from build123d import *

# Parameters (mm, degrees)
F1_DEPTH = 19
F3_DEPTH = 4


with BuildPart() as f1:
    # F0 (on Right) → F1 (new body)
    with BuildSketch(Plane.YZ):
        Polygon((6.931424, 163.453436), (-53.068576, 163.453436), (-115.068576, 5.453436), (-115.068576, -134.546564), (68.931424, -134.546564), (68.931424, 5.453436), align=None)
    extrude(amount=F1_DEPTH)

    # F2 (on face) → F3 (cut)
    with BuildSketch(Plane.YZ.offset(19)):
        Polygon((-5.074208, 131.790936), (-45.087915, 132.872388), (-45.087915, 77.357873), (-5.074208, 77.357873), align=None)
    extrude(amount=-F3_DEPTH, mode=Mode.SUBTRACT)


solid = f1.part
Here's how the part is built. I have some questions about the finished solid (model axes, mm). Coordinates: 2 decimals unless noted, no trailing zeros. Write each loop counter-clockwise with the first axis right and the second up, starting at its lowest first coordinate (ties: lowest second). Pieces come first, ordered by that corner, then holes.
Item 1: If I drill on line 1 (X direction, y = -16.5, z = 83); line 2 (Y direction, x = 7.25, z = 41); line 3 (Y direction, x = 3.75, z = 95), over which ranges is the centre line in solid material (lowest first)?
Item 2: I want a section at C-C on y = -25. Write out the boundary of the cut face in (x, z), and give its area (3 significant figures).
Item 3: I want a section at B-B on x = 10. Write out the boundary of the cut face in (y, z).
Item 4: Will these pins go through, and if not, where does the flat tip stop? pin 1 (20 mm diameter, centred on y = -22, z = 106.5, fed in from +X); pin 2 (4.5 mm diameter, centred on x = 16.5, z = 101, fed in from -Y); pin 3 (4 mm diameter, centred on x = 10.5, z = 110.5, fed in from -Y).
Item 5: If we mould it in two halves opening along Y, with no side actions, what happens to faces 1 (the flat face through (9, 68.931, -66)), 2 (the flat face through (9, -23, 163.453)), 3 (the flat face through (15, -25, 106))? For each: +Y half, -Y half, draft (parallel to the pull), parting line (faces both ways), or undercut.
Item 6: I want a section at D-D on z = 27.5. Write out the boundary of the cut face in (x, y), and give its area (3 significant figures).
Item 7: I want a section at A-A on z = 101.5. Write out the boundary of the cut face in (x, y).
Findings below:
1. line 1: x = 0 to 15
1. line 2: y = -101.12 to 54.98
1. line 3: y = -79.93 to 33.79
2. outline: (0, -134.55) - (19, -134.55) - (19, 77.36) - (15, 77.36) - (15, 132.33) - (19, 132.33) - (19, 163.45) - (0, 163.45) - close
2. area: 5,440 mm2
3. outline: (-115.07, -134.55) - (68.93, -134.55) - (68.93, 5.45) - (6.93, 163.45) - (-53.07, 163.45) - (-115.07, 5.45) - close
4. pin 1: stops at x = 15
4. pin 2: stops at y = -78.46
4. pin 3: stops at y = -74.63
5. face 1: +Y half
5. face 2: draft
5. face 3: undercut
6. outline: (0, -106.42) - (19, -106.42) - (19, 60.28) - (0, 60.28) - close
6. area: 3,170 mm2
7. outline: (0, -77.38) - (19, -77.38) - (19, -45.09) - (15, -45.09) - (15, -5.07) - (19, -5.07) - (19, 31.24) - (0, 31.24) - close
